Model file for the job. Use its own axes, mm. A direction names the side the tool comes from. Give positions to 0.01 mm unless a question says otherwise; leave off trailing zeros. Write each loop counter-clockwise with the first axis right and the second up, starting at its lowest first coordinate (ties: lowest second). Pieces come first, ordered by that corner, then holes.
```python
from build123d import *

# Parameters (mm, degrees)
F0_R      = 10
F1_DEPTH  = 20
F2_R      = 2.5
F3_DEPTH  = 5
F13_DEPTH = 20.001
F4_R      = 1
F6_DEPTH  = 20.001
F9_R      = 5.3210242514
F10_DEPTH = 25


# Not quite as in the source:
# - the program builds the solid bodies; features that only make, move or delete a surface that nothing else refers to are left out


with BuildPart() as f1:
    # F0 (on Front) → F1 (new body)
    with BuildSketch(Plane.XZ):
        Circle(F0_R)
    extrude(amount=F1_DEPTH)

    # F2 (on face) → F3 (cut)
    with BuildSketch(Plane.XZ.offset(20)):
        Circle(F2_R)
    extrude(amount=-F3_DEPTH, mode=Mode.SUBTRACT)

    # F12 (on face) → F13 (cut, through all)
    with BuildSketch(Plane.XZ.offset(20)):
        with BuildLine():
            ThreePointArc((2.7924241272, 9.6022063868), (1.4103077913, 9.9000521177), (0, 10))
            Line((0, 10), (0, 5))
            ThreePointArc((0, 5), (0.7051538957, 4.9500260589), (1.3962120636, 4.8011031934))
            Line((1.3962120636, 4.8011031934), (2.7924241272, 9.6022063868))
        make_face()
        with BuildLine():
            Line((0, 5), (0, 10))
            ThreePointArc((0, 10), (-1.4103077913, 9.9000521177), (-2.7924241272, 9.6022063868))
            Line((-2.7924241272, 9.6022063868), (-1.3962120636, 4.8011031934))
            ThreePointArc((-1.3962120636, 4.8011031934), (-0.7051538957, 4.9500260589), (0, 5))
        make_face()
    extrude(amount=-F13_DEPTH, mode=Mode.SUBTRACT)

    # F4
    f4_edges = [f1.edges().sort_by_distance(p)[0] for p in [
        (-2.792424, -10, 9.602206),
        (2.792424, -10, 9.602206),
        (-1.396212, -10, 4.801103),
        (1.396212, -10, 4.801103),
    ]]
    fillet(f4_edges, radius=F4_R)

    # F5 (on face) → F6 (cut, through all)
    with BuildSketch(Plane.XZ.offset(20)):
        Polygon((8.2990381057, 0.75), (7, 1.5), (5.7009618943, 0.75), (5.7009618943, -0.75), (7, -1.5), (8.2990381057, -0.75), align=None)
    extrude(amount=-F6_DEPTH, mode=Mode.SUBTRACT)

    # F9 (on face) → F10 (cut)
    with BuildSketch(Plane(origin=(0, 0, 0), x_dir=(-1, 0, 0), z_dir=(0, 1, 0))):
        with Locations((11.770372279, -20.3817021102)):
            Circle(F9_R)
    extrude(amount=-F10_DEPTH, mode=Mode.SUBTRACT)


solid = f1.part
```
1. Probe probe 1 along Y at (x, z) = (-1, 0.5); probe 2 along X at (y, z) = (-3.5, 5.75); probe 3 along Z at (x, y) = (2.75, -12.25). List the from-to ranges inside material, lowest first.
Calculated:
probe 1: y = -15 to 0
probe 2: x = -8.18 to -1.67, 1.67 to 8.18
probe 3: z = -9.61 to 9.02
2. Slice it at A-A, the plane z = 0. Write the cut outline in (x, y).
Calculated:
outline: (-10, -20) - (-2.5, -20) - (-2.5, -15) - (2.5, -15) - (2.5, -20) - (5.7, -20) - (5.7, 0) - (-10, 0) - close; (8.3, -20) - (10, -20) - (10, 0) - (8.3, 0) - close
3. Which spindle directions (+Z, -Z, +X, -X, +Y, -Y) get a long thin tool onto all of the face, cutting with end or side? Do faces 1 (the flat face through (0, -15, 0)), 2 (the flat face through (2, -20, -2)), 3 (the flat face through (6.36, -10.14, 1.13)), 4 (the flat face through (-2.08, -10.14, 7.15)). Say none if no direction does.
Calculated:
face 1: -Y
face 2: +Z, -Z, +X, -X, -Y
face 3: +Y, -Y
face 4: +Z, +Y, -Y
4. Pull direction Z, two halves, no side cores. Call faces 5 (the flat face through (8.299, -10, 0)), 6 (the cylindrical face through (3, -9.9, 9.2)), 7 (the flat face through (5.701, -10, 0)), 8 (the flat face through (0, 0, 0)): +Z half, -Z half, draft (parallel to the pull), parting line (faces both ways), or undercut.
Calculated:
face 5: undercut
face 6: +Z half
face 7: undercut
face 8: draft
5. Slice it at D-D, the plane y = -4.25. Write the cut outline in (x, z), and give its area (3 significant figures).
Calculated:
outline: (-3.84, 9.23) arc R10 ccw (long way) to (3.84, 9.23) arc R1 ccw to (2.5, 8.59) - (1.65, 5.68) arc R1 cw to (0.58, 4.97) arc R5 ccw to (-0.58, 4.97) arc R1 cw to (-1.65, 5.68) - (-2.5, 8.59) arc R1 ccw to start; hole (5.7, -0.75) - (7, -1.5) - (8.3, -0.75) - (8.3, 0.75) - (7, 1.5) - (5.7, 0.75) - close
area: 287 mm2
6. Pin check, flat tips, straight feed: P1, Ø1, axis at y = -17, z = 2.5, coming from the -X side; P2, Ø4, axis at y = -12, z = -5.5, coming from the +X side; P3, Ø8, axis at x = -5, y = -11.5, coming from the -Z side. Stop position of each tip, or through.
Calculated:
P1: stops at x = -9.8
P2: stops at x = 9.37
P3: stops at z = -9.95
7. Slice it at B-B, the plane y = -17.75. Write the cut outline in (x, z).
Calculated:
outline: (-3.84, 9.23) arc R10 ccw (long way) to (3.84, 9.23) arc R1 ccw to (2.5, 8.59) - (1.65, 5.68) arc R1 cw to (0.58, 4.97) arc R5 ccw to (-0.58, 4.97) arc R1 cw to (-1.65, 5.68) - (-2.5, 8.59) arc R1 ccw to start; hole circle Ø5 at (0, 0); hole (5.7, -0.75) - (7, -1.5) - (8.3, -0.75) - (8.3, 0.75) - (7, 1.5) - (5.7, 0.75) - close
8. Slice it at C-C, the plane x = 6.25. Write the cut outline in (y, z), and give its area (3 significant figures).
Calculated:
outline: (-20, -7.81) - (0, -7.81) - (0, -1.07) - (-20, -1.07) - close; (-20, 1.07) - (0, 1.07) - (0, 7.81) - (-20, 7.81) - close
area: 270 mm2
